Build history of the part. All positions in model axes, mm. A direction names the side the tool comes from. Give positions to 0.01 mm unless a question says otherwise; leave off trailing zeros. Order: outer loops, then holes, each group sorted by start corner. A loop starts at its lowest first (then second) coordinate and runs counter-clockwise, first axis right, second up. Notation, with made-up numbers: (5.5, 74.5) - (27.5, 74.5) arc R27 ccw to (27.5, 106.5) - close; hole circle Ø2 at (7, 83.5). An arc over 180 degrees is marked (long way). Use a Markdown table: item, result.
from build123d import *

# Parameters (mm, degrees)
SKETCH1_W                  = 2.54
SKETCH1_H                  = 2.54
SKETCH1_W_2                = 0.65
SKETCH1_H_2                = 0.65
BOSS_EXTRUDE1_DEPTH        = 14.1
CHAMFER1_SIZE              = 0.5
SKETCH4_W                  = 1.6
SKETCH4_H                  = 1.6
CUT_EXTRUDE2_DEPTH         = 1.5
CUT_EXTRUDE1_START         = -10.2
SKETCH2_W                  = 1.6
SKETCH2_H                  = 1.6
CUT_EXTRUDE1_DEPTH         = 10.2
BOSS_EXTRUDE2_DEPTH        = 0.05
SKETCH5_W                  = 0.2
SKETCH5_H                  = 3.3
CUT_EXTRUDE3_DEPTH         = 0.47
LPATTERN1_COUNT            = 5
LPATTERN1_PITCH            = 2.54
CHAMFER1_OF_LPATTERN1_SIZE = 0.5


with BuildPart() as part:
    # Sketch1 → Boss-Extrude1 (new body)
    with BuildSketch(Plane.XY):
        with Locations((1.27, 1.27)):
            Rectangle(SKETCH1_W, SKETCH1_H)
        with Locations((1.27, 1.27)):
            Rectangle(SKETCH1_W_2, SKETCH1_H_2, mode=Mode.SUBTRACT)
    boss_extrude1 = extrude(amount=BOSS_EXTRUDE1_DEPTH)

    # Chamfer1
    chamfer1_edges = [part.edges().sort_by_distance(p)[0] for p in [
        (1.595, 1.27, 0),
        (1.27, 1.595, 0),
        (0.945, 1.27, 0),
        (1.27, 0.945, 0),
    ]]
    chamfer(chamfer1_edges, length=CHAMFER1_SIZE)

    # Sketch4 → Cut-Extrude2 (cut)
    with BuildSketch(Plane(origin=(0, 2.54, 0), x_dir=(1, 0, 0), z_dir=(0, 1, 0))):
        with Locations((1.27, -4.7)):
            Rectangle(SKETCH4_W, SKETCH4_H)
    cut_extrude2 = extrude(amount=-CUT_EXTRUDE2_DEPTH, mode=Mode.SUBTRACT)

    # Sketch2 → Cut-Extrude1 (cut)
    with BuildSketch(Plane.XY.offset(14.1).offset(CUT_EXTRUDE1_START)):
        with Locations((1.27, 1.27)):
            Rectangle(SKETCH2_W, SKETCH2_H)
    cut_extrude1 = extrude(amount=CUT_EXTRUDE1_DEPTH, mode=Mode.SUBTRACT)

    # Sketch3 → Boss-Extrude2 (add)
    with BuildSketch(Plane(origin=(0, 2.54, 0), x_dir=(1, 0, 0), z_dir=(0, 1, 0))):
        Polygon((2.12, -3.5), (0.42, -3.5), (1.27, -1.75), align=None)
    extrude(amount=BOSS_EXTRUDE2_DEPTH)

    # Sketch5 → Cut-Extrude3 (cut)
    with BuildSketch(Plane(origin=(0, 2.54, 0), x_dir=(1, 0, 0), z_dir=(0, 1, 0))):
        with Locations((0.57, -7.15)):
            Rectangle(SKETCH5_W, SKETCH5_H)
        with Locations((1.97, -7.15)):
            Rectangle(SKETCH5_W, SKETCH5_H)
    cut_extrude3 = extrude(amount=-CUT_EXTRUDE3_DEPTH, mode=Mode.SUBTRACT)

    # LPattern1: Boss-Extrude1, Cut-Extrude2, Cut-Extrude1, Cut-Extrude3 ×5
    with Locations(*[(i * LPATTERN1_PITCH, 0, 0) for i in range(1, LPATTERN1_COUNT)]):
        add(boss_extrude1)
        add(cut_extrude2, mode=Mode.SUBTRACT)
        add(cut_extrude1, mode=Mode.SUBTRACT)
        add(cut_extrude3, mode=Mode.SUBTRACT)

    # Chamfer1 of LPattern1
    chamfer1_of_lpattern1_edges = [part.edges().sort_by_distance(p)[0] for p in [
        (4.135, 1.27, 0),
        (3.81, 1.595, 0),
        (3.485, 1.27, 0),
        (3.81, 0.945, 0),
        (6.675, 1.27, 0),
        (6.35, 1.595, 0),
        (6.025, 1.27, 0),
        (6.35, 0.945, 0),
        (9.215, 1.27, 0),
        (8.89, 1.595, 0),
        (8.565, 1.27, 0),
        (8.89, 0.945, 0),
        (11.755, 1.27, 0),
        (11.43, 1.595, 0),
        (11.105, 1.27, 0),
        (11.43, 0.945, 0),
    ]]
    chamfer(chamfer1_of_lpattern1_edges, length=CHAMFER1_OF_LPATTERN1_SIZE)


solid = part.part
1) Slice it at C-C (y = 1.1). State how many separate pieces and enclosed holes the cut face has, and give its area (3 significant figures).
Computed:
| item | result |
|---|---|
| separate pieces | 6 |
| enclosed holes | 0 |
| area | 83.5 mm² |
2) Wall check: line 1 (X direction, y = 1.4, z = 11.5); line 2 (Y direction, x = 1, z = 7.75); line 3 (Z direction, x = 1.75, y = 2.3). Give the ranges that are in metal, low to high. Write a range as from..to.
Computed:
| item | result |
|---|---|
| line 1 | x = 0..0.47, 2.07..3.01, 4.61..5.55, 7.15..8.09, 9.69..10.63, 12.23..12.7 |
| line 2 | y = 0..0.47, 2.07..2.54 |
| line 3 | z = 0..3.9, 5.5..14.1 |
3) Two-plate mould, pull along Y, no slides. Class faces 4 (the flat face through (4, 2, 3.9)), 5 (the flat face through (1, 2.59, 3)), 6 (the flat face through (1, 2.07, 10)): +Y half, -Y half, draft (parallel to the pull), parting line (faces both ways), or undercut.
Computed:
| item | result |
|---|---|
| face 4 | draft |
| face 5 | +Y half |
| face 6 | undercut |
4) Slice it at A-A (x = 11.5). Write the cut outline in (y, z) (3 decimals).
Computed:
| item | result |
|---|---|
| outline | (0, 0) - (0.445, 0) - (0.945, 0.5) - (0.945, 3.9) - (0.47, 3.9) - (0.47, 14.1) - (0, 14.1) - close; (1.595, 0.5) - (2.095, 0) - (2.54, 0) - (2.54, 3.9) - (1.595, 3.9) - close; (2.07, 5.5) - (2.54, 5.5) - (2.54, 14.1) - (2.07, 14.1) - close |
5) Pin check, flat tip, straight feed: P1, Ø0.5, axis at x = 6.5, z = 9.5, coming from the +Y side. Stop position of the tip, or through.
Computed:
| item | result |
|---|---|
| P1 | stops at y = 2.54 |
6) Tool access for faces 1 (the flat face through (12.7, 1, 7)), 2 (the flat face through (9, 2, 3.9)), 3 (the flat face through (4, 2.07, 10)): list every direction of +Z, -Z, +X, -X, +Y, -Y with a clear straight run to the whole face (end or side of a thin tool).
Computed:
| item | result |
|---|---|
| face 1 | +Z, -Z, +X, +Y, -Y |
| face 2 | +Y |
| face 3 | +Z |
7) Slice it at B-B (z = 11.5). Write the cut outline in (x, y), and give its area (3 significant figures).
Computed:
| item | result |
|---|---|
| outline | (0, 0) - (12.7, 0) - (12.7, 2.54) - (0, 2.54) - close; hole (0.47, 0.47) - (2.07, 0.47) - (2.07, 2.07) - (0.47, 2.07) - close; hole (3.01, 0.47) - (4.61, 0.47) - (4.61, 2.07) - (3.01, 2.07) - close; hole (5.55, 0.47) - (7.15, 0.47) - (7.15, 2.07) - (5.55, 2.07) - close; hole (8.09, 0.47) - (9.69, 0.47) - (9.69, 2.07) - (8.09, 2.07) - close; hole (10.63, 0.47) - (12.23, 0.47) - (12.23, 2.07) - (10.63, 2.07) - close |
| area | 19.5 mm² |
8) Slice it at D-D (z = 4.5). Write the cut outline in (x, y), and give its area (3 significant figures).
Computed:
| item | result |
|---|---|
| outline | (0, 0) - (12.7, 0) - (12.7, 2.54) - (12.23, 2.54) - (12.23, 0.47) - (10.63, 0.47) - (10.63, 2.54) - (9.69, 2.54) - (9.69, 0.47) - (8.09, 0.47) - (8.09, 2.54) - (7.15, 2.54) - (7.15, 0.47) - (5.55, 0.47) - (5.55, 2.54) - (4.61, 2.54) - (4.61, 0.47) - (3.01, 0.47) - (3.01, 2.54) - (2.07, 2.54) - (2.07, 0.47) - (0.47, 0.47) - (0.47, 2.54) - (0, 2.54) - close |
| area | 15.7 mm² |
